For this review, take the finished solid that the model builds, in its own axes (mm). Give positions to 0.01 mm unless a question says otherwise; leave off trailing zeros. Write each loop counter-clockwise with the first axis right and the second up, starting at its lowest first coordinate (ties: lowest second). Pieces come first, ordered by that corner, then holes. Notation, with made-up numbers: (73, 72) -> (83, 72) arc R14 cw to (83, 99) -> close; hole circle Ø10 at (-13.75, 72). An arc over 180 degrees is marked (long way). Return JSON: item names as keys, results as strings.
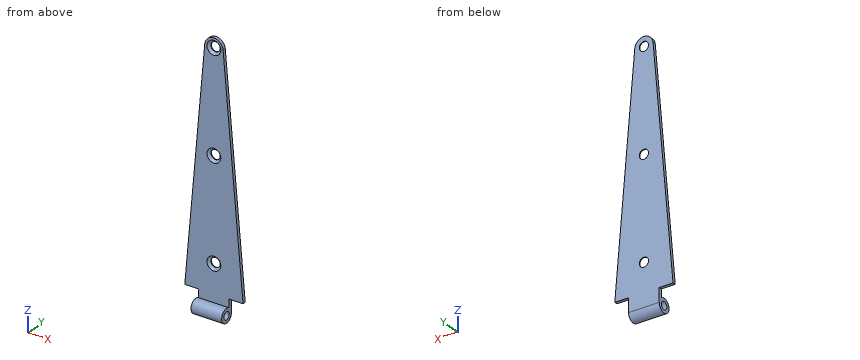
from build123d import *

# Parameters (mm, degrees)
F1_DEPTH       = 5.08
F2_W           = 50.8
F2_H           = 5.08
F3_DEPTH       = 22.86
F4_W           = 50.8
F4_H           = 5.08
F6_R           = 15.24
F8_D           = 15.24
F8_CSINK_D     = 22.86
F8_CSINK_ANGLE = 90


with BuildPart() as f1:
    # F0 (on Front) → F1 (new body)
    with BuildSketch(Plane.XZ):
        Polygon((48.26, 551.614324), (0, 0), (96.52, 0), align=None)
    extrude(amount=F1_DEPTH)

    # F2 (on face) → F3 (join)
    with BuildSketch(Plane(origin=(0, 0, 0), x_dir=(1, 0, 0), z_dir=(0, 0, -1))):
        with Locations((48.26, 2.54)):
            Rectangle(F2_W, F2_H)
    extrude(amount=F3_DEPTH)

    # F4 (on face) → F5 (revolve)
    with BuildSketch(Plane(origin=(0, 0, -22.86), x_dir=(1, 0, 0), z_dir=(0, 0, -1))):
        with Locations((48.26, 2.54)):
            Rectangle(F4_W, F4_H)
    revolve(axis=Axis((35.56, -11.43, -22.86), (1, 0, 0)))

    # F6
    f6_edges = [f1.edges().sort_by_distance(p)[0] for p in [
        (48.26, -2.54, 551.614324),
    ]]
    fillet(f6_edges, radius=F6_R)

    # F8 (through all)
    with Locations(Plane.XZ.offset(5.08)):
        with Locations((48.26, 46.554934), (48.26, 211.654934), (48.26, 376.754934)):
            CounterSinkHole(F8_D / 2, F8_CSINK_D / 2, counter_sink_angle=F8_CSINK_ANGLE)


solid = f1.part
1. Add section B-B, the plane y = -11.43. State the section outline as (x, z) points.
Results found:
{"outline": "(22.86, -34.29) -> (73.66, -34.29) -> (73.66, -29.21) -> (22.86, -29.21) -> close; (22.86, -16.51) -> (73.66, -16.51) -> (73.66, -11.43) -> (22.86, -11.43) -> close"}
2. Add section A-A, the plane x = 48.26. State the section outline as (y, z) points, plus the area to 3 significant figures.
Results found:
{"outline": "(-5.08, -13.36) arc R11.43 ccw (long way) to (0, -22.86) -> (0, 38.93) -> (-1.27, 38.93) -> (-5.08, 35.12) -> close; (-5.08, 57.98) -> (-1.27, 54.17) -> (0, 54.17) -> (0, 204.03) -> (-1.27, 204.03) -> (-5.08, 200.22) -> close; (-5.08, 223.08) -> (-1.27, 219.27) -> (0, 219.27) -> (0, 369.13) -> (-1.27, 369.13) -> (-5.08, 365.32) -> close; (-5.08, 388.18) -> (-1.27, 384.37) -> (0, 384.37) -> (0, 391.99) -> (-5.08, 391.99) -> close; hole circle Ø12.7 at (-11.43, -22.86)", "area": "2,080 mm²"}
3. Add section D-D, the plane z = 97. State the section outline as (x, y) points.
Results found:
{"outline": "(8.49, -5.08) -> (88.03, -5.08) -> (88.03, 0) -> (8.49, 0) -> close"}
4. Add section C-C, the plane x = 85.5. State the section outline as (y, z) points.
Results found:
{"outline": "(-5.08, 0) -> (0, 0) -> (0, 125.96) -> (-5.08, 125.96) -> close"}
5. To check wall thickness, follow probe 1 along Z at (x, y) = (48.5, -11.43); probe 2 along Y at (x, z) = (50.5, -12.5); probe 3 along Y at (x, z) = (12.5, 139). State the ranges of each line that lie inside material, in increasing order.
Results found:
{"probe 1": "z = -34.29 to -29.21, -16.51 to -11.43", "probe 2": "y = -16.26 to -6.6, -5.08 to 0", "probe 3": "y = -5.08 to 0"}
6. For pin 1 (4 mm diameter, centred on x = 6.5, y = -3, fed in from -Z); pin 2 (5 mm diameter, centred on x = 25, z = 201.5, fed in from -Y); pin 3 (12 mm diameter, centred on y = -3.5, z = 49, fed in from -X); pin 4 (3 mm diameter, centred on y = -7.5, z = 334.5, fed in from -X), all flat-tipped, find the tip position at first contact; note any pin that passes through.
Results found:
{"pin 1": "stops at z = 0", "pin 2": "stops at y = -5.08", "pin 3": "stops at x = 3.76", "pin 4": "passes through"}
